Autodesk Inventor part; units mm, degrees
ref_plane "YZ Plane" through (0, 0, 0) normal (1, 0, 0) x (0, 1, 0)
ref_plane "XZ Plane" through (0, 0, 0) normal (0, 1, 0) x (-1, 0, 0)
ref_plane "XY Plane" through (0, 0, 0) normal (0, 0, 1) x (1, 0, 0)
sketch "Sketch2" plane through (0, 0, 0) normal (0, 0, 1) x (1, 0, 0)
  line L0 (-13, -7.5) -> (13, -7.5)
  line L1 (13, -7.5) -> (13, 7.5)
  line L2 (13, 7.5) -> (-13, 7.5)
  line L3 (-13, 7.5) -> (-13, -7.5)
  line L4 (-13, -7.5) -> (13, 7.5) construction
  line L5 (13, -7.5) -> (-13, 7.5) construction
  line L6 (-13, 2) -> (-10, 2)
  line L7 (-10, 2) -> (-10, -2)
  line L8 (-10, -2) -> (-13, -2)
  line L9 (0, 7.5) -> (0, -7.5) construction
  line L10 (13, -2) -> (10, -2)
  line L11 (10, -2) -> (10, 2)
  line L12 (10, 2) -> (13, 2)
  point P0 (0, 0)
  point P1 (0, 0)
  point P2 (-10, 0)
  point P3 (10, 0)
  dimension "d0" = 26
  dimension "d3" = 15
  dimension "d7" = 4
  dimension "d17" = 3
extrude "Extrusion1" add sketch "Sketch2" along normal mid plane 4
sketch "Sketch3" plane through (0, 0, -2) normal (0, 0, -1) x (-1, 0, 0)
  line L0 (-13, -7.5) -> (13, -7.5)
  line L1 (13, -7.5) -> (13, 7.5)
  line L2 (13, 7.5) -> (-13, 7.5)
  line L3 (-13, 7.5) -> (-13, -7.5)
  line L4 (-10, 5.5) -> (10, 5.5)
  line L5 (10, -5.5) -> (-10, -5.5)
  line L6 (-10, 5.5) -> (-10, -5.5)
  line L7 (10, 5.5) -> (10, -5.5)
  point P0 (0, 0)
  dimension "d4" = 2
  dimension "d18" = 2
  dimension "d19" = 3
  dimension "d20" = 3
extrude "Extrusion2" cut sketch "Sketch3" against normal blind 2 contours L4 L7 L5 L6
extrude "Extrusion3" add sketch "Sketch2" along normal blind 2 and the other way blind 12 contours L3 L6 L7 L8 | L10 L11 L12 L1
sketch "Sketch4" plane through (13, 2, 2) normal (0, 1, 0) x (1, 0, 0)
  line L0 (-3, 4.007) -> (-3, 14)
  arc A0 (-3, 14) -> (-3, 11.4019) centre (-2.25, 12.701) ccw
  line L1 (-3, 11.4019) -> (-3, 14)
  line L2 (-13, 2) -> (-13, 0) construction
  line L3 (-26, 0) -> (0, 0) construction
  line L4 (-23, 14) -> (-23, 4.007)
  arc A1 (-23, 11.4019) -> (-23, 14) centre (-23.75, 12.701) ccw
  line L5 (-3, 4) -> (-3, 14)
  dimension "d13" = 1.5
  dimension "d14" = 0.75
extrude "Extrusion4" add sketch "Sketch4" against normal blind 4
equation "\"d18\" = d4"
equation "\"d20\" = d19"
properties part number "Cover"
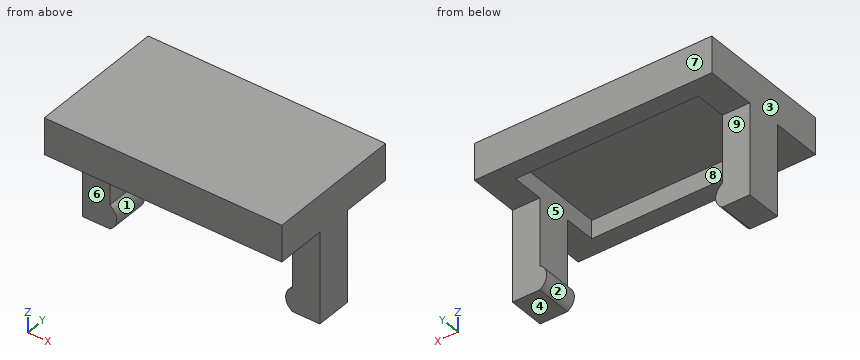
Geometry: final body of the model. Coordinates: model frame, mm. Face numbers are marked on the shaded views. A direction names the side the tool comes from. Round coordinates to 2 decimals unless told otherwise and drop trailing zeros. Order: outer loops, then holes, each group sorted by start corner. A loop starts at its lowest first (then second) coordinate and runs counter-clockwise, first axis right, second up. Notation, with made-up numbers: (35, 39.5) - (70, 39.5) arc R13 ccw to (70, 43.5) - close; hole circle Ø8 at (18, 29.5). An arc over 180 degrees is marked (long way). Write item = value, one per line. Start each with the question number.
Q1. Pull-direction query (Z, two-part tool) for the marked faces 1, 2, 3 and 4; classes: +Z half, -Z half, draft (parallel to the pull), parting line (faces both ways), or undercut.
Q2. Cut plane D-D on y = 6. Return the cut outline in (x, z).
Q3. Cut plane B-B on y = -3. Return the cut outline in (x, z), and give its area (3 significant figures).
Q4. Cut plane C-C on x = -7.75. Return the cut outline in (y, z), and give its area (3 significant figures).
Q5. Ray query, line 1 (Z direction, x = -8.5, y = -3.25); line 2 (Z direction, x = 8.75, y = -6.5). Return the intervals inside material, ascending. Write a range as from..to.
Q6. Access query for the marked faces 5, 6, 7, 8 and 9. Directions: +Z, -Z, +X, -X, +Y, -Y. A direction counts if a zero-diameter tool reaches every point of the face in a straight line with its end or side. Return the directions, or none.
Q7. Pin query (flat end, axial travel): pin 1 (1.9 mm diameter, centred on x = 11.5, z = -6, fed in from -Y); pin 2 (1.6 mm diameter, centred on x = -3, y = -4, fed in from -Z); pin 3 (6 mm diameter, centred on x = 2.5, z = -3.5, fed in from -Y); pin 4 (4 mm diameter, centred on x = -11, z = -8, fed in from +Y). Return the tip coordinate at first contact, or that it passes through.
Q8. Cut plane A-A on z = -7.75. Return the cut outline in (x, y).
Outcome:
q1.face_1 = undercut
q1.face_2 = undercut
q1.face_3 = draft
q1.face_4 = -Z half
q2.outline = (-13, -2) - (13, -2) - (13, 2) - (-13, 2) - close
q3.outline = (-13, -2) - (-10, -2) - (-10, 0) - (10, 0) - (10, -2) - (13, -2) - (13, 2) - (-13, 2) - close
q3.area = 64.0 mm^2
q4.outline = (-7.5, -2) - (-5.5, -2) - (-5.5, 0) - (5.5, 0) - (5.5, -2) - (7.5, -2) - (7.5, 2) - (-7.5, 2) - close
q4.area = 38.0 mm^2
q5.line_1 = 0..2
q5.line_2 = -2..2
q6.face_5 = none
q6.face_6 = -Z, +X, -X, -Y
q6.face_7 = +Z, -Z, +X, -X, +Y
q6.face_8 = -Z
q6.face_9 = -Z, +X, -X, +Y
q7.pin_1 = -2
q7.pin_2 = 0
q7.pin_3 = -7.5
q7.pin_4 = 2
q8.outline = (-13, -2) - (-10, -2) - (-10, 2) - (-13, 2) - close; (10, -2) - (13, -2) - (13, 2) - (10, 2) - close
